Can you work these out from the drawing? Everything is in mm from the part's minimum corner. A direction names the side the tool comes from. Round coordinates to 2 decimals unless told otherwise and drop trailing zeros. Write each loop counter-clockwise with the first axis right and the second up, starting at its lowest first coordinate (ties: lowest second). Pieces come first, ordered by that corner, then holes. Notation, with made-up numbers: (16, 65.5) - (48, 65.5) arc R8 cw to (48, 72.5) - close; hole circle Ø8 at (75, -22.75). An arc over 180 degrees is marked (long way). One line per item, written item: value. Start each with the question number.
(1) I want a section at C-C on z = 6.75. List the corners of the cut face in (x, y) for me.
(2) I want a section at B-B on z = 17.25. List the corners of the cut face in (x, y) for me, plus the area to 3 significant figures.
(3) On a 3-axis mill with a long thin cutter (end or side, diameter ignored), from which of +Z, -Z, +X, -X, +Y, -Y can I reach the whole of each face in a straight line? I mean the marked faces 1 and 2. Say none if no direction works.
(4) I want a section at A-A on y = 5.35. List the corners of the cut face in (x, z) for me, plus the area to 3 significant figures.
(5) I'm going to push flat-ended pins straight in: pin 1 Ø1.1 at (x, y) = (0.5, 2) entering from -Z; pin 2 Ø1.5 at (y, z) = (7, 3) entering from +X. Where does each tip first touch, or does it pass through?
(6) If I drill on L1, parallel to X at y = 1.75, z = 25.5; L2, parallel to X at y = 5.5, z = 7; L3, parallel to Z at x = 51.5, y = 4.75, over which ranges is the centre line in solid material (lowest first)? Write a range as from..to.
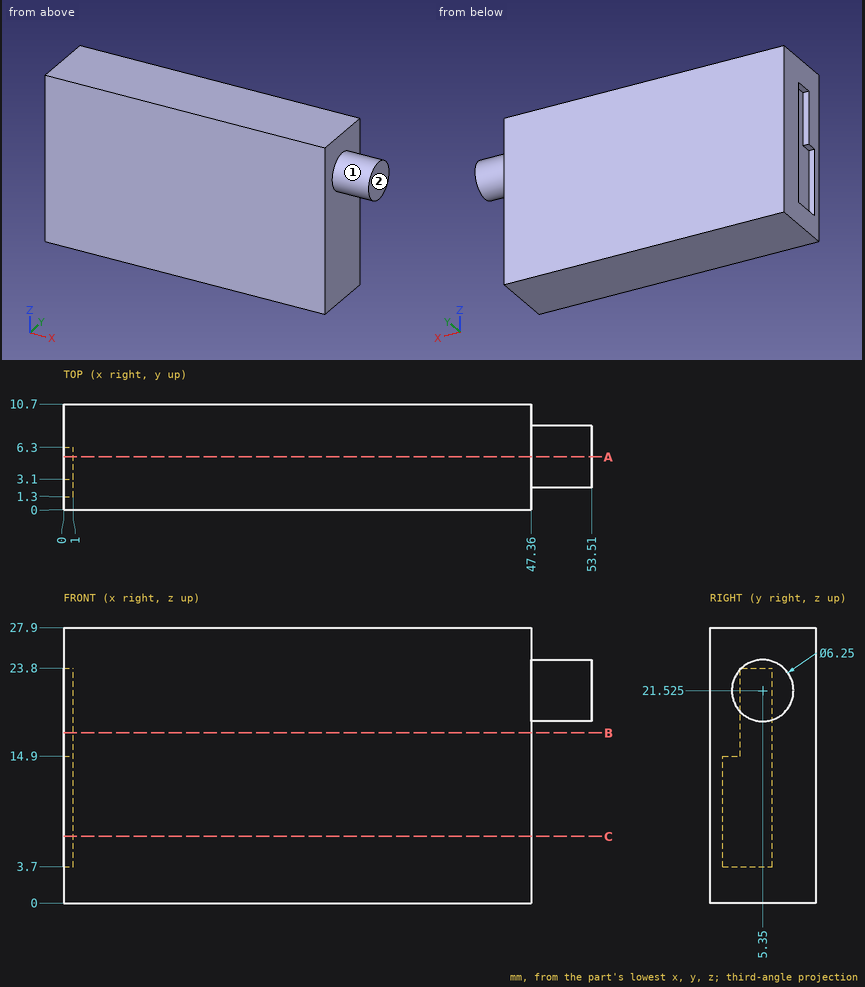
Established:
1. outline: (0, 0) - (47.36, 0) - (47.36, 10.7) - (0, 10.7) - (0, 6.3) - (1, 6.3) - (1, 1.3) - (0, 1.3) - close
2. outline: (0, 0) - (47.36, 0) - (47.36, 10.7) - (0, 10.7) - (0, 6.3) - (1, 6.3) - (1, 3.1) - (0, 3.1) - close
2. area: 504 mm2
3. face 1: +X
3. face 2: +Z, -Z, +X, +Y, -Y
4. outline: (0, 0) - (47.36, 0) - (47.36, 18.4) - (53.51, 18.4) - (53.51, 24.65) - (47.36, 24.65) - (47.36, 27.9) - (0, 27.9) - (0, 23.8) - (1, 23.8) - (1, 3.7) - (0, 3.7) - close
4. area: 1,340 mm2
5. pin 1: z = 0
5. pin 2: x = 47.36
6. L1: 0..47.36
6. L2: 1..47.36
6. L3: 18.46..24.59
